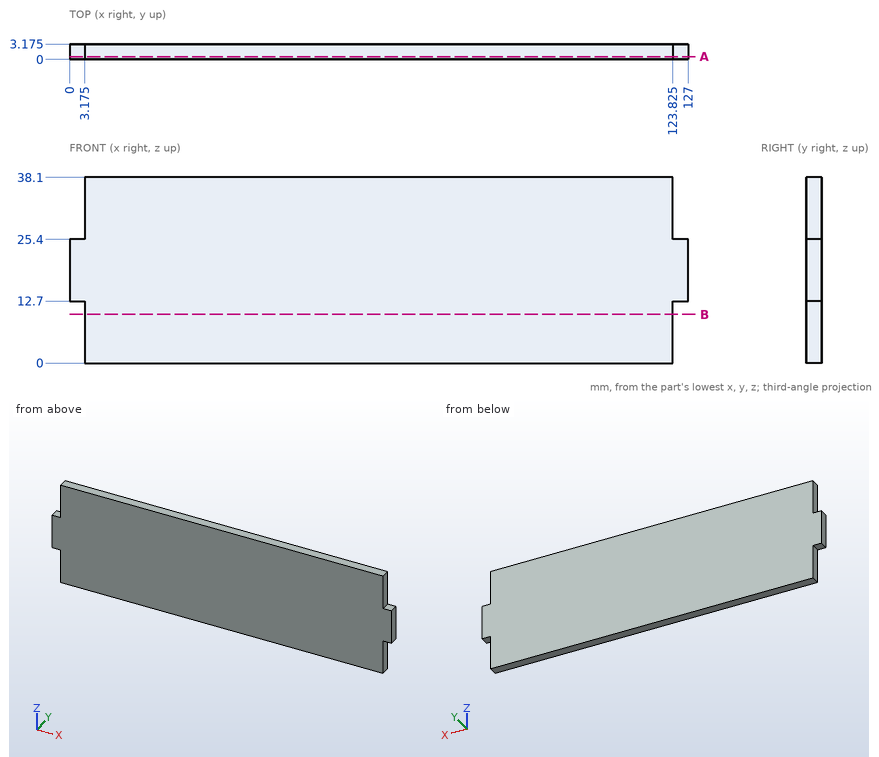
For this review, use the dimensioned drawing (mm, ordinates from the lowest corner) and the shaded views. Coordinates: 2 decimals unless noted, no trailing zeros. Order: outer loops, then holes, each group sorted by start corner. A loop starts at its lowest first (then second) coordinate and runs counter-clockwise, first axis right, second up. Notation, with made-up numbers: (14, -19.5) - (65, -19.5) arc R16 ccw to (65, 0.5) - close; hole circle Ø9 at (-7, 71.5). An arc over 180 degrees is marked (long way). Answer as a JSON object with one key per item and string values. Group by question number.
1. We need section B-B on z = 10. State the section outline as (x, y) points (3 decimals).
2. We need section A-A on y = 0.6. State the section outline as (x, z) points (3 decimals).
3. For probe 1 along X at (y, z) = (2.9, 4) (3 decimals), list the stretches that pass through material, from the lowest coordinate up.
4. Clearance check with flat-ended pins moving along their axes: P1, Ø1.6, axis at x = 1, y = 1.5, coming from the +Z side; P2, Ø1, axis at x = 1.5, y = 1.5, coming from the -Z side; P3, Ø1.6, axis at y = 1, z = 5.5, coming from the +X side (3 decimals). State where each tip first meets the part, or that it passes through.
Final values:
{
 "1": {"outline": "(3.175, 0) - (123.825, 0) - (123.825, 3.175) - (3.175, 3.175) - close"},
 "2": {"outline": "(0, 12.7) - (3.175, 12.7) - (3.175, 0) - (123.825, 0) - (123.825, 12.7) - (127, 12.7) - (127, 25.4) - (123.825, 25.4) - (123.825, 38.1) - (3.175, 38.1) - (3.175, 25.4) - (0, 25.4) - close"},
 "3": {"probe 1": "3.175 to 123.825"},
 "4": {"P1": "z = 25.4", "P2": "z = 12.7", "P3": "x = 123.825"}
}
